from build123d import *

# Parameters (mm, degrees)
SKETCH1_R                    = 56.769
SKETCH1_R_2                  = 30.1625
BOSS_EXTRUDE1_DEPTH          = 17.272
SKETCH2_R                    = 31.877
CUT_EXTRUDE1_DEPTH           = 7.747
CHAMFER1_SIZE                = 0.762
SKETCH4_R                    = 4.2164
CUT_EXTRUDE2_DEPTH           = 18.272
CHAMFER2_SIZE                = 0.381
CIRPATTERN1_COUNT            = 8
CHAMFER2_OF_CIRPATTERN1_SIZE = 0.381
CUT_EXTRUDE3_DEPTH           = 0.79375


with BuildPart() as part:
    # Sketch1 → Boss-Extrude1 (new body)
    with BuildSketch(Plane(origin=(0, 0, 0), x_dir=(1, 0, 0), z_dir=(0, 1, 0))):
        Circle(SKETCH1_R)
        Circle(SKETCH1_R_2, mode=Mode.SUBTRACT)
    extrude(amount=BOSS_EXTRUDE1_DEPTH)

    # Sketch2 → Cut-Extrude1 (cut)
    with BuildSketch(Plane(origin=(0, 17.272, 0), x_dir=(1, 0, 0), z_dir=(0, 1, 0))):
        Circle(SKETCH2_R)
    extrude(amount=-CUT_EXTRUDE1_DEPTH, mode=Mode.SUBTRACT)

    # Chamfer1
    chamfer1_edges = [part.edges().sort_by_distance(p)[0] for p in [
        (-31.877, 17.272, 0),
        (-56.769, 0, 0),
        (-56.769, 17.272, 0),
    ]]
    chamfer(chamfer1_edges, length=CHAMFER1_SIZE)

    # Sketch5 → Cut-Revolve1 (revolve, cut)
    with BuildSketch(Plane.XY):
        Polygon((-41.275, 0), (-41.275, 1.6256), (-38.608, 0.6604), (-38.608, 1.27), (0, 1.27), (0, 0), align=None)
    revolve(axis=Axis((0, 17.272, 0), (0, -1, 0)), mode=Mode.SUBTRACT)

    # Sketch4 → Cut-Extrude2 (cut, through all)
    with BuildSketch(Plane(origin=(0, 17.272, 0), x_dir=(1, 0, 0), z_dir=(0, 1, 0))):
        with Locations((-17.632368756, 42.568303788)):
            Circle(SKETCH4_R)
    cut_extrude2 = extrude(amount=-CUT_EXTRUDE2_DEPTH, mode=Mode.SUBTRACT)

    # Chamfer2
    chamfer2_edges = [part.edges().sort_by_distance(p)[0] for p in [
        (-21.848768756, 0, -42.568303788),
        (-21.848768756, 17.272, -42.568303788),
    ]]
    chamfer(chamfer2_edges, length=CHAMFER2_SIZE)

    # CirPattern1: Cut-Extrude2 ×8 about axis
    cirpattern1_axis = Axis((0, 0, 0), (0, 1, 0))
    for i in range(1, CIRPATTERN1_COUNT):
        add(cut_extrude2.rotate(cirpattern1_axis, i * 360 / CIRPATTERN1_COUNT), mode=Mode.SUBTRACT)

    # Chamfer2 of CirPattern1
    chamfer2_of_cirpattern1_edges = [part.edges().sort_by_distance(p)[0] for p in [
        (-45.54974882, 0, -14.650923724),
        (-45.54974882, 17.272, -14.650923724),
        (-42.568303788, 0, 21.848768756),
        (-42.568303788, 17.272, 21.848768756),
        (-14.650923724, 0, 45.54974882),
        (-14.650923724, 17.272, 45.54974882),
        (21.848768756, 0, 42.568303788),
        (21.848768756, 17.272, 42.568303788),
        (45.54974882, 0, 14.650923724),
        (45.54974882, 17.272, 14.650923724),
        (42.568303788, 0, -21.848768756),
        (42.568303788, 17.272, -21.848768756),
        (14.650923724, 0, -45.54974882),
        (14.650923724, 17.272, -45.54974882),
    ]]
    chamfer(chamfer2_of_cirpattern1_edges, length=CHAMFER2_OF_CIRPATTERN1_SIZE)

    # Sketch6 → Cut-Extrude3 (cut, symmetric)
    with BuildSketch(Plane.XY):
        Polygon((-40.64, 0.933144104), (-56.769, 1.778429176), (-56.769, -1.196708046), (-40.64, -1.196708046), align=None)
        Polygon((56.769, 1.645313417), (56.769, -1.196708046), (40.64, -1.196708046), (40.64, 0.800028345), align=None)
    extrude(amount=CUT_EXTRUDE3_DEPTH, both=True, mode=Mode.SUBTRACT)


solid = part.part
CAD build for the part. Positions are in the model's coordinates, mm. A direction names the side the tool comes from. Coordinates: 2 decimals unless noted, no trailing zeros. Loops run counter-clockwise (first coordinate to the right, second up) from the corner with the lowest first, then second, coordinate; pieces in that order, holes last. Notation, with made-up numbers: (26.5, 39) - (57.5, 39) arc R11 cw to (57.5, 58) - close; hole circle Ø6 at (6.5, 66.25). An arc over 180 degrees is marked (long way). Write item = value, one per line. Start each with the question number.
Q1. Flat gauge pins, fed straight in: pin 1 Ø1.3 at (x, y) = (49.5, 1) entering from +Z; pin 2 Ø1 at (y, z) = (6.5, 14.5) entering from -X; pin 3 Ø0.9 at (x, y) = (-51, 1) entering from -Z. Where does each tip first touch, or does it go through?
Q2. Which spindle directions (+Z, -Z, +X, -X, +Y, -Y) get a long thin tool onto all of the face, cutting with end or side? Do faces 4 (the flat face through (-1, 0, 46)), 5 (the cylindrical face through (30.405, 13.066, -9.575)). Say none if no direction does.
Q3. Cut at A-A, the plane x = 0. List the corners of the cut face in (y, z) (1 decimal), then the cut area to 3 significant figures.
Q4. Cut at B-B, the plane y = 6.75. Give the number of separate pieces and of enclosed holes in the cut face, then the cut area to 3 significant figures.
Q5. Pull direction X, two halves, no side cores. Call faces 1 (the conical face through (15, 17, 46)), 2 (the conical face through (-1.223, 0.122, 56.115)), 3 (the flat face through (24, 17.272, 24)): pulls with the +X half, pulls with the -X half, needs draft (parallel to the pull), parting line crosses it, or undercut.
Q6. Drill centre lines: L1, parallel to X at y = 13.5, z = 0; L2, parallel to Z at x = -40, y = 10; L3, parallel to Y at x = 10, z = -35. Where is each one in solid material? Low to high.
Computed:
q1.pin_1 = 28.92
q1.pin_2 = -55.02
q1.pin_3 = -25.83
q2.face_4 = +Z, -Z, +X, -X, -Y
q2.face_5 = +Y
q3.outline = (0, -56) - (0.8, -56.8) - (16.5, -56.8) - (17.3, -56) - (17.3, -32.6) - (16.5, -31.9) - (9.5, -31.9) - (9.5, -30.2) - (1.3, -30.2) - (1.3, -38.6) - (0.7, -38.6) - (1.6, -41.3) - (0, -41.3) - close; (0, 41.3) - (1.6, 41.3) - (0.7, 38.6) - (1.3, 38.6) - (1.3, 30.2) - (9.5, 30.2) - (9.5, 31.9) - (16.5, 31.9) - (17.3, 32.6) - (17.3, 56) - (16.5, 56.8) - (0.8, 56.8) - (0, 56) - close
q3.area = 863 mm²
q4.separate_pieces = 1
q4.enclosed_holes = 9
q4.area = 6,820 mm²
q5.face_1 = undercut
q5.face_2 = parting line crosses it
q5.face_3 = needs draft
q6.L1 = -56.77 to -31.88, 31.88 to 56.77
q6.L2 = -40.28 to -20.98, -14.29 to 14.29, 20.98 to 40.28
q6.L3 = 1.27 to 17.27
